Source: CAD feature listing. Evaluate the final solid. Frame: model axes, mm. A direction names the side the tool comes from. Give positions to 0.01 mm unless a question says otherwise; leave off trailing zeros. Loops run counter-clockwise (first coordinate to the right, second up) from the corner with the lowest first, then second, coordinate; pieces in that order, holes last. Notation, with made-up numbers: M 67.5,-11.5 L 77.5,-11.5 A17 cw 77.5,11.5 Z; hole C 4,16 d6. An arc over 180 degrees is marked long. Answer in a Markdown table with one row per item.
```python
from build123d import *

# Parameters (mm, degrees)
F3_DEPTH = 100
F5_D     = 10


with BuildPart() as f1:
    # F0 (on Right) → F1 (revolve)
    with BuildSketch(Plane.YZ):
        with BuildLine():
            Line((0, 32.3266497701), (0, 0))
            Line((0, 0), (9, 0))
            Line((9, 0), (13.925663583, 20.3266497701))
            Line((13.925663583, 20.3266497701), (25, 20.3266497701))
            Line((25, 20.3266497701), (25, 26.3266497701))
            add(Edge.make_bspline(
                [(25, 26.3266497701), (25, 32.3266497701), (0, 32.3266497701)],
                knots=[0, 0, 0, 1.5707963268, 1.5707963268, 1.5707963268], degree=2, weights=[1, 0.7071067812, 1]))
        make_face()
    revolve(axis=Axis((0, 0, 16.1633248851), (0, 0, -1)))

    # F2 (on Top) → F3 (intersect)
    with BuildSketch(Plane.XY):
        with BuildLine():
            ThreePointArc((-3.754235732, 22.3323114682), (-11.041772693, 11.1341950684), (-22.4685130723, 4.2106403335))
            ThreePointArc((-22.4685130723, 4.2106403335), (-25.5082976179, 0.022874934), (-22.51186286, -4.1960168477))
            ThreePointArc((-22.51186286, -4.1960168477), (-11.2684741638, -11.1275544115), (-4.0917559502, -22.2160492621))
            ThreePointArc((-4.0917559502, -22.2160492621), (0.0139431693, -25.0707596903), (4.1012988558, -22.1898465746))
            ThreePointArc((4.1012988558, -22.1898465746), (11.1616155781, -11.1006865584), (22.2852773965, -4.0948540004))
            ThreePointArc((22.2852773965, -4.0948540004), (25.1766523938, 0.0226602251), (22.2424904136, 4.1097944591))
            ThreePointArc((22.2424904136, 4.1097944591), (10.9343752254, 11.1089431069), (3.7628862808, 22.3085545833))
            ThreePointArc((3.7628862808, 22.3085545833), (0.0126414158, 24.9518154629), (-3.754235732, 22.3323114682))
        make_face()
    extrude(amount=F3_DEPTH, mode=Mode.INTERSECT)

    # F5 (through all)
    with Locations(Plane(origin=(0, 0, 0), x_dir=(1, 0, 0), z_dir=(0, 0, -1))):
        with Locations((0, 0)):
            Hole(F5_D / 2)


solid = f1.part
```
1) Material intervals for L1, parallel to Y at x = 0, z = 19; L2, parallel to Y at x = 0, z = 11; L3, parallel to Z at x = -14.5, y = -6, sorted ascending.
Reply:
| item | result |
|---|---|
| L1 | y = -13.6 to -5, 5 to 13.6 |
| L2 | y = -11.67 to -5, 5 to 11.67 |
| L3 | z = 20.33 to 31 |
2) Section A-A, the plane z = 24.5. Return loops of the section in (x, y), then the cut area to 3 significant figures.
Reply:
| item | result |
|---|---|
| outline | M -24.9,-2.24 A4.44 ccw -22.51,-4.2 A30 cw -4.09,-22.22 A4.36 ccw -0.86,-24.99 A25 ccw 0.86,-24.99 A4.36 ccw 4.1,-22.19 A30 cw 22.29,-4.09 A4.35 ccw 24.96,-1.34 A25 ccw 24.96,1.34 A4.35 ccw 22.24,4.11 A30 cw 3.76,22.31 A4 ccw -3.75,22.33 A30 cw -22.47,4.21 A4.44 ccw -24.9,2.24 A25 ccw Z; hole C 0,0 d10 |
| area | 1,110 mm² |
3) Section B-B, the plane z = 6.5. Return loops of the section in (x, y), then the cut area to 3 significant figures.
Reply:
| item | result |
|---|---|
| outline | C 0,0 d21.15; hole C 0,0 d10 |
| area | 273 mm² |
4) Set-up query: faces 1 (the flat face through (9, -11, 20.327)), 2 (the cylindrical face through (-2.86, -24, 23.6)). Return all of +Z, -Z, +X, -X, +Y, -Y with unobstructed straight access to the full face (end or side cutting, diameter ignored); none if empty.
Reply:
| item | result |
|---|---|
| face 1 | -Z |
| face 2 | +Z, -Z, -X, -Y |
5) Pull-direction query (X, two-part tool) for faces 3 (the flat face through (-4, -4, 0)), 4 (the cylindrical face through (1.08, 4.88, 16.33)), 5 (the conical face through (3.289, 10.444, 8.047)), 6 (the cylindrical face through (-10.907, 11.266, 25.589)); classes: released by +X, released by -X, zero draft, split by the parting line, or undercut.
Reply:
| item | result |
|---|---|
| face 3 | zero draft |
| face 4 | undercut |
| face 5 | split by the parting line |
| face 6 | released by -X |
6) Pin query (flat end, axial travel): pin 1 Ø1 at (x, z) = (-18.5, 25) entering from -Y; pin 2 Ø3 at (x, z) = (14, 10) entering from +Y; pin 3 Ø5 at (x, y) = (-14, -11.5) entering from -Z; pin 4 Ø1.5 at (y, z) = (-1.5, 19) entering from +X. Return the tip coordinate at first contact, or that it passes through.
Reply:
| item | result |
|---|---|
| pin 1 | stops at y = -6.17 |
| pin 2 | passes through |
| pin 3 | stops at z = 20.33 |
| pin 4 | stops at x = 13.72 |
